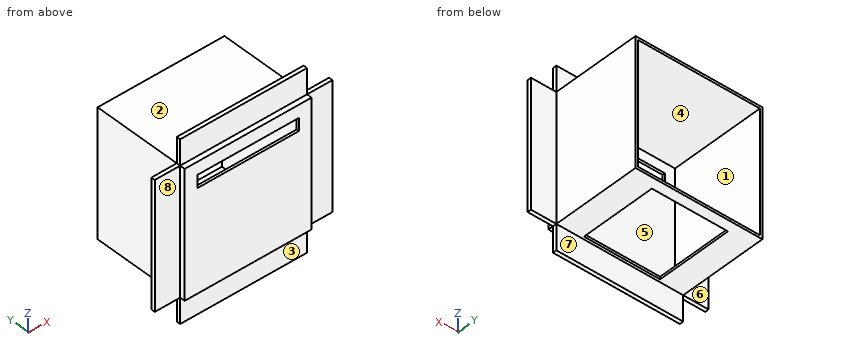
```python
from build123d import *

# Parameters (mm, degrees)
SKETCH1_W                = 20
SKETCH1_H                = 100
BOSS_EXTRUDE1_DEPTH      = 3
BOSS_EXTRUDE2_DEPTH      = 70
BOSS_EXTRUDE2_DEPTH_BACK = 7
SKETCH2_W                = 100
SKETCH2_H                = 100
SHELL1_START             = -2
SHELL1_OUTLINE_W         = 96
SHELL1_OUTLINE_H         = 96
SHELL1_DEPTH             = 75
SKETCH3_W                = 80
SKETCH3_H                = 10
CUT_EXTRUDE1_DEPTH       = 11
SKETCH6_W                = 60
SKETCH6_H                = 60
CUT_EXTRUDE2_DEPTH       = 2


# Read off the part's stored shape, not the designer's step: Shell1
with BuildPart() as part:
    # Sketch1 → Boss-Extrude1 (new body)
    with BuildSketch(Plane(origin=(0, 0, 0), x_dir=(1, 0, 0), z_dir=(0, 1, 0))):
        Polygon((0, 50), (-50, 50), (-50, -50), (0, -50), (50, -50), (50, 0), (50, 50), align=None)
        with Locations((-60, 0)):
            Rectangle(SKETCH1_W, SKETCH1_H)
        Polygon((0, -50), (-50, -50), (-50, -70), (0, -70), (50, -70), (50, -50), align=None)
        Polygon((70, 50), (50, 50), (50, 0), (50, -50), (70, -50), (70, 0), align=None)
        Polygon((-50, 70), (-50, 50), (0, 50), (50, 50), (50, 70), (0, 70), align=None)
    extrude(amount=BOSS_EXTRUDE1_DEPTH)

    # Sketch2 → Boss-Extrude2 (add, two sides: drawn at the far end of the back side and taken through both)
    with BuildSketch(Plane(origin=(0, 3, 0), x_dir=(-1, 0, 0), z_dir=(0, 1, 0)).offset(-BOSS_EXTRUDE2_DEPTH_BACK)):
        Rectangle(SKETCH2_W, SKETCH2_H)
    extrude(amount=BOSS_EXTRUDE2_DEPTH + BOSS_EXTRUDE2_DEPTH_BACK)

    # Shell1 outline → Shell1 (cut)
    with BuildSketch(Plane(origin=(0, 0, 0), x_dir=(1, 0, 0), z_dir=(0, 1, 0)).offset(SHELL1_START)):
        Rectangle(SHELL1_OUTLINE_W, SHELL1_OUTLINE_H)
    extrude(amount=SHELL1_DEPTH, mode=Mode.SUBTRACT)

    # Sketch3 → Cut-Extrude1 (cut)
    with BuildSketch(Plane.XZ.offset(4)):
        with Locations((0, 35)):
            Rectangle(SKETCH3_W, SKETCH3_H)
    extrude(amount=-CUT_EXTRUDE1_DEPTH, mode=Mode.SUBTRACT)

    # Sketch6 → Cut-Extrude2 (cut)
    with BuildSketch(Plane(origin=(0, 0, -50), x_dir=(-1, 0, 0), z_dir=(0, 0, -1))):
        with Locations((0, 35)):
            Rectangle(SKETCH6_W, SKETCH6_H)
    extrude(amount=-CUT_EXTRUDE2_DEPTH, mode=Mode.SUBTRACT)


solid = part.part
```
Part model, mm, in its own coordinate system. Face numbers are marked on the shaded views. A direction names the side the tool comes from. Round coordinates to 2 decimals unless told otherwise and drop trailing zeros. Loops run counter-clockwise (first coordinate to the right, second up) from the corner with the lowest first, then second, coordinate; pieces in that order, holes last.
Item 1: Cut at D-D, the plane y = 18. Give the cut face in (x, z), then the cut area to 3 significant figures.
Item 2: Cut at B-B, the plane z = 14.5. Give the cut face in (x, y), then the cut area to 3 significant figures.
Item 3: Drop flat-ended pins along their axis: P1, Ø5, axis at x = -22, y = 36.5, coming from the -Z side; P2, Ø2, axis at x = -4, y = -3, coming from the +Z side; P3, Ø5, axis at y = 27.5, z = -22.5, coming from the -X side; P4, Ø22, axis at x = -22, z = 56, coming from the +Y side. Give the stop position or say it passes through.
Item 4: Cut at A-A, the plane x = -34. Give the cut face in (y, z), then the cut area to 3 significant figures.
Item 5: Cut at C-C, the plane z = 32.5. Give the cut face in (x, y), then the cut area to 3 significant figures.
Item 6: Mould opens along Z. For the marked faces 1, 2, 3 and 4 say: +Z half, -Z half, draft (parallel to the pull), parting line (faces both ways), or undercut.
Item 7: Drill centre lines: line 1 (Z direction, x = 34.5, y = 55.5); line 2 (Y direction, x = 45, z = 23). Where is each one in solid material? Low to high.
Item 8: 3-axis set-ups, long thin cutter, end or side, ignore diameter. For the marked faces 5, 6, 7 and 8: which of +Z, -Z, +X, -X, +Y, -Y reach the whole face in a straight line?
A:
1. outline: (-50, -50) - (-30, -50) - (-30, -48) - (-48, -48) - (-48, 48) - (48, 48) - (48, -48) - (30, -48) - (30, -50) - (50, -50) - (50, 50) - (-50, 50) - close
1. area: 664 mm2
2. outline: (-70, 0) - (-50, 0) - (-50, -4) - (50, -4) - (50, 0) - (70, 0) - (70, 3) - (50, 3) - (50, 73) - (48, 73) - (48, -2) - (-48, -2) - (-48, 73) - (-50, 73) - (-50, 3) - (-70, 3) - close
2. area: 620 mm2
3. P1: stops at z = 48
3. P2: stops at z = 50
3. P3: stops at x = -50
3. P4: stops at y = 73
4. outline: (-4, -50) - (0, -50) - (0, -70) - (3, -70) - (3, -50) - (73, -50) - (73, -48) - (-2, -48) - (-2, 30) - (-4, 30) - close; (-4, 40) - (-2, 40) - (-2, 48) - (73, 48) - (73, 50) - (3, 50) - (3, 70) - (0, 70) - (0, 50) - (-4, 50) - close
4. area: 600 mm2
5. outline: (-70, 0) - (-50, 0) - (-50, -4) - (-40, -4) - (-40, -2) - (-48, -2) - (-48, 73) - (-50, 73) - (-50, 3) - (-70, 3) - close; (40, -4) - (50, -4) - (50, 0) - (70, 0) - (70, 3) - (50, 3) - (50, 73) - (48, 73) - (48, -2) - (40, -2) - close
5. area: 460 mm2
6. face 1: undercut
6. face 2: +Z half
6. face 3: draft
6. face 4: undercut
7. line 1: z = -50 to -48, 48 to 50
7. line 2: y = -4 to -2
8. face 5: +Y
8. face 6: +Z, -Z, -X, +Y
8. face 7: -Z, +X, -X, +Y
8. face 8: +Z, -Z, -X, -Y
